from build123d import *

# Parameters (mm, degrees)
F0_W     = 18
F0_H     = 17.850996
F0_W_2   = 14
F0_H_2   = 13.850996
F1_DEPTH = 10
F2_W     = 18
F2_H     = 25
F3_DEPTH = 2
F4_R     = 5
F5_R     = 1


with BuildPart() as f1:
    # F0 (on Top) → F1 (new body)
    with BuildSketch(Plane.XY):
        Rectangle(F0_W, F0_H)
        Rectangle(F0_W_2, F0_H_2, mode=Mode.SUBTRACT)
    extrude(amount=F1_DEPTH)

    # F2 (on Top) → F3 (join)
    with BuildSketch(Plane.XY):
        with Locations((0, -3.574502)):
            Rectangle(F2_W, F2_H)
    extrude(amount=F3_DEPTH)

    # F4
    f4_edges = [f1.edges().sort_by_distance(p)[0] for p in [
        (9, -16.074502, 1),
        (-9, -16.074502, 1),
    ]]
    fillet(f4_edges, radius=F4_R)

    # F5
    f5_edges = [f1.edges().sort_by_distance(p)[0] for p in [
        (9, -8.925498, 6),
        (-9, -8.925498, 6),
        (-9, 8.925498, 5),
        (9, 8.925498, 5),
    ]]
    fillet(f5_edges, radius=F5_R)


solid = f1.part
Here's how the part is built. I have some questions about the finished solid (model axes, mm). A direction names the side the tool comes from. Give positions to 0.01 mm unless a question says otherwise; leave off trailing zeros. Order: outer loops, then holes, each group sorted by start corner. A loop starts at its lowest first (then second) coordinate and runs counter-clockwise, first axis right, second up. Notation, with made-up numbers: (-12.5, 38.5) -> (36.5, 38.5) arc R33 cw to (36.5, 77.5) -> close; hole circle Ø8 at (54, 9). An arc over 180 degrees is marked (long way). One line per item, written item: value. Start each with the question number.
1. Imagine slicing it at A-A, the plane z = 4.75. List the corners of the cut face in (x, y) for me.
2. Imagine slicing it at D-D, the plane x = -6. List the corners of the cut face in (y, z) for me.
3. For faces 1 (the face through (8.7, -8.64, 6.06)), 2 (the face through (7, 0, 6)), 3 (the face through (-8.715, -8.625, 6.056)), which set-ups out of +Z, -Z, +X, -X, +Y, -Y let a thin tool reach every point of the face, with its end or its side?
4. Imagine slicing it at C-C, the plane z = 1.5. List the corners of the cut face in (x, y) for me, plus the area to 3 significant figures.
5. Will these pins go through, and if not, where does the flat tip stop? pin 1 Ø9 at (x, y) = (1, -13) entering from +Z; pin 2 Ø2.5 at (x, z) = (-2, 5.5) entering from -Y; pin 3 Ø5 at (x, y) = (-2, -0.5) entering from +Z.
6. We'd pull the mould along X, two halves only. Please class faces 4 (the face through (9, 0, 5)), 5 (the face through (-7, 0, 6)), 6 (the face through (0, -8.925, 6)): released by +X, released by -X, zero draft, split by the parting line, or undercut.
7. Imagine slicing it at B-B, the plane y = 1.5. List the corners of the cut face in (x, z) for me, plus the area to 3 significant figures.
8. I need wall thicknesses on probe 1 along Y at (x, z) = (6.5, 9.25); probe 2 along X at (y, z) = (5.75, 3); probe 3 along Z at (x, y) = (7.75, -9). Which ranges of each line are inside material? Lowest first, please. Write a range as from..to.
Values follow:
1. outline: (-9, -7.93) arc R1 ccw to (-8, -8.93) -> (8, -8.93) arc R1 ccw to (9, -7.93) -> (9, 7.93) arc R1 ccw to (8, 8.93) -> (-8, 8.93) arc R1 ccw to (-9, 7.93) -> close; hole (-7, -6.93) -> (7, -6.93) -> (7, 6.93) -> (-7, 6.93) -> close
2. outline: (-15.66, 0) -> (8.93, 0) -> (8.93, 10) -> (6.93, 10) -> (6.93, 2) -> (-6.93, 2) -> (-6.93, 10) -> (-8.93, 10) -> (-8.93, 2) -> (-15.66, 2) -> close
3. face 1: +Z, +X, -Y
3. face 2: +Z
3. face 3: +Z, -X, -Y
4. outline: (-9, -11.07) arc R5 ccw to (-4, -16.07) -> (4, -16.07) arc R5 ccw to (9, -11.07) -> (9, 7.93) arc R1 ccw to (8, 8.93) -> (-8, 8.93) arc R1 ccw to (-9, 7.93) -> close
4. area: 439 mm2
5. pin 1: stops at z = 10
5. pin 2: stops at y = -8.93
5. pin 3: stops at z = 2
6. face 4: released by +X
6. face 5: undercut
6. face 6: zero draft
7. outline: (-9, 0) -> (9, 0) -> (9, 10) -> (7, 10) -> (7, 2) -> (-7, 2) -> (-7, 10) -> (-9, 10) -> close
7. area: 68.0 mm2
8. probe 1: y = -8.93..-6.93, 6.93..8.93
8. probe 2: x = -9..-7, 7..9
8. probe 3: z = 0..2
